Could you check a few things on this model? Use its own coordinates, in mm. A direction names the side the tool comes from. Give positions to 0.01 mm unless a question says otherwise; leave off trailing zeros. Loops run counter-clockwise (first coordinate to the right, second up) from the corner with the lowest first, then second, coordinate; pieces in that order, holes last. Notation, with made-up numbers: (-17.75, 80.25) - (20.25, 80.25) arc R12 ccw to (20.25, 89.25) - close; hole circle Ø9 at (54.25, 83). An arc over 180 degrees is marked (long way). Answer in a Markdown table with one row per item. Add a question column.
Autodesk Inventor part; units mm, degrees
ref_plane "作業平面1" through (0, 0, 1.4) normal (0, 0, 1) x (1, 0, 0)
ref_plane "作業平面2" through (0, 0, 1) normal (0, 0, -1) x (-1, 0, 0)
ref_plane "作業平面3" through (0, 0, 1.5) normal (0, 0, -1) x (-1, 0, 0)
sketch "スケッチ1" plane through (0, 0, 0) normal (0, 0, 1) x (1, 0, 0)
  circle A0 centre (0, 0) radius 3
  circle A1 centre (0, 0) radius 3.5
  circle A2 centre (0, 0) radius 5
  circle A3 centre (0, 0) radius 4.5
  dimension "d0" = 6
  dimension "d1" = 7
  dimension "d2" = 10
  dimension "d3" = 9
extrude "押し出し1" add sketch "スケッチ1" along normal blind 2.4
sketch "スケッチ2" plane through (0, 0, 2.4) normal (0, 0, 1) x (1, 0, 0)
  point P0 (0, 0)
ref_plane "作業平面1" through (0, 0, 1.4) normal (0, 0, 1) x (1, 0, 0)
ref_plane "作業平面2" through (0, 0, 1) normal (0, 0, -1) x (-1, 0, 0)
ref_plane "作業平面3" through (0, 0, 1.5) normal (0, 0, -1) x (-1, 0, 0)
sketch "スケッチ3" plane through (0, 0, 1.5) normal (0, 0, -1) x (-1, 0, 0)
  circle A0 centre (0, 4) radius 0.5
  circle A1 centre (0, 0) radius 4.5
  circle A2 centre (0, 0) radius 3.5
  line L0 (0, 4.5) -> (0, 3.5)
revolve "回転1" add sketch "スケッチ3" angle 360 about axis through (0, 4.5, 1.5) along (0, -1, 0) picked at (0.0723, 4.1502) contours A0 L0
pattern_circular "円形状パターン1" count 8 over 360 about axis through (0, 0, -10) along (0, 0, 1) of "回転1"
sketch "スケッチ4" plane through (0, 0, 1) normal (0, 0, -1) x (-1, 0, 0)
  circle A0 centre (0, 0) radius 3.5
  circle A1 centre (0, 0) radius 4.5
extrude "押し出し2" add sketch "スケッチ4" along normal blind 0.5
sketch "スケッチ5" plane through (0, 0, 1.4) normal (0, 0, 1) x (1, 0, 0)
  circle A0 centre (0, 0) radius 3.5
  circle A1 centre (0, 0) radius 4.5
extrude "押し出し3" add sketch "スケッチ5" along normal blind 0.5
sketch "スケッチ6" plane through (0, 0, 0) normal (0, 0, -1) x (-1, 0, 0)
  circle A0 centre (0, 0) radius 3
  circle A1 centre (0, 0) radius 5.6
  dimension "d17" = 11.2
  dimension "d20" = 6
extrude "押し出し4" add sketch "スケッチ6" along normal blind 0.6
sketch "スケッチ7" plane through (0, 0, 0) normal (0, 0, -1) x (-1, 0, 0)
  point P0 (0, 0)
properties part number "φ6φ10ベアリング" material "鋼 AISI 1006 85 HR"
(1) On a 3-axis mill with a long thin cutter (end or side, diameter ignored), from which of +Z, -Z, +X, -X, +Y, -Y can I reach the whole of each face in a straight line? I mean faces 4 (the flat face through (0, -4, 0)), 5 (the cylindrical face through (5.595, -0.246, -0.296)), 6 (the flat face through (2, 5, 0)). Say none if no direction works.
(2) Please list where these lines run through material, in increasing order: line 1 (Z direction, x = -3.5, y = 1.5); line 2 (Y direction, x = 0, z = 2.2); line 3 (Y direction, x = 0, z = 1.8).
(3) For pin 1 Ø1.5 at (y, z) = (2.5, 1) entering from -X; pin 2 Ø2.5 at (x, y) = (1.5, -2) entering from +Z; pin 3 Ø3 at (x, y) = (-1, 0) entering from +Z, each with a flat end and sliding along its axis, tell me the tip position at first contact or that it passes through.
(4) We'd pull the mould along Y, two halves only. Please class faces 1 (the cylindrical face through (-1.08, 4.88, 1.18)), 2 (the cylindrical face through (3.233, 1.341, 0.246)), 3 (the flat face through (-2.4, -2.4, -0.6)): pulls with the +Y half, pulls with the -Y half, needs draft (parallel to the pull), parting line crosses it, or undercut.
(5) I want a section at B-B on z = 1.15. State how many separate pieces and enclosed holes the cut face has, then the cut area to 3 significant figures.
(6) I want a section at A-A on z = 0.25. Please give me the cut outline in (x, y), then the cut area to 3 significant figures.
Reported:
| question | item | result |
|---|---|---|
| 1 | face 4 | none |
| 1 | face 5 | +Z, -Z |
| 1 | face 6 | +Z |
| 2 | line 1 | -0.6 to 0, 0.5 to 1, 1.4 to 1.9 |
| 2 | line 2 | -5 to -4.5, -3.5 to -3, 3 to 3.5, 4.5 to 5 |
| 2 | line 3 | -5 to -3, 3 to 5 |
| 3 | pin 1 | x = -4.68 |
| 3 | pin 2 | z = 2.4 |
| 3 | pin 3 | through |
| 4 | face 1 | parting line crosses it |
| 4 | face 2 | undercut |
| 4 | face 3 | needs draft |
| 5 | separate pieces | 10 |
| 5 | enclosed holes | 2 |
| 5 | area | 28.3 mm² |
| 6 | outline | circle Ø10 at (0, 0); circle Ø7 at (0, 0); hole circle Ø9 at (0, 0); hole circle Ø6 at (0, 0) |
| 6 | area | 25.1 mm² |
